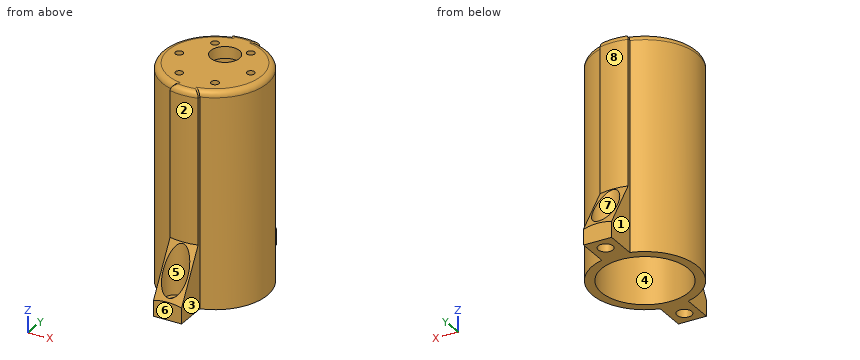
from build123d import *

# Parameters (mm, degrees)
F1_R      = 3.15
F2_DEPTH  = 92
F3_R      = 18.6
F5_DEPTH  = 87
F4_R      = 6.15
F4_R_2    = 1.65
F8_DEPTH  = 92.0010001
F9_R      = 5.25
F10_DEPTH = 87
F11_R     = 2.5


with BuildPart() as f2:
    # F1 (on Top) → F2 (new body)
    with BuildSketch(Plane.XY):
        with BuildLine():
            Line((6, 35.2), (-6, 35.2))
            Line((-6, 35.2), (-6, 21.6852484422))
            ThreePointArc((-6, 21.6852484422), (0, 22.5), (6, 21.6852484422))
            Line((6, 21.6852484422), (6, 35.2))
        make_face()
        with Locations((0, 29.2)):
            Circle(F1_R, mode=Mode.SUBTRACT)
        with BuildLine():
            ThreePointArc((6, 21.6852484422), (0, 22.5), (-6, 21.6852484422))
            ThreePointArc((-6, 21.6852484422), (-22.5, 0), (-6, -21.6852484422))
            ThreePointArc((-6, -21.6852484422), (0, -22.5), (6, -21.6852484422))
            ThreePointArc((6, -21.6852484422), (17.9060045795, -13.6244265934), (22.5, 0))
            ThreePointArc((22.5, 0), (17.9060045795, 13.6244265934), (6, 21.6852484422))
        make_face()
        with BuildLine():
            ThreePointArc((6, -21.6852484422), (0, -22.5), (-6, -21.6852484422))
            Line((-6, -21.6852484422), (-6, -35.2))
            Line((-6, -35.2), (6, -35.2))
            Line((6, -35.2), (6, -21.6852484422))
        make_face()
        with Locations((0, -29.2)):
            Circle(F1_R, mode=Mode.SUBTRACT)
    extrude(amount=F2_DEPTH)

    # F3 (on face) → F5 (cut)
    with BuildSketch(Plane(origin=(0, 0, 0), x_dir=(1, 0, 0), z_dir=(0, 0, -1))):
        Circle(F3_R)
    extrude(amount=-F5_DEPTH, mode=Mode.SUBTRACT)

    # F6 (on Right) → F7 (revolve, cut)
    with BuildSketch(Plane.YZ):
        Polygon((36.6852484422, 102), (23.6852484422, 102), (23.6852484422, 27.5166604984), (36.6852484422, 5), align=None)
    revolve(axis=Axis((0, 0, 51.2388907373), (0, 0, 1)), mode=Mode.SUBTRACT)

    # F4 (on face) → F8 (cut, through all)
    with BuildSketch(Plane.XY.offset(92)):
        with Locations((0, 7.5)):
            Circle(F4_R)
        with Locations((-15.3, 0)):
            Circle(F4_R_2)
        with Locations((-7.65, -13.2501886779)):
            Circle(F4_R_2)
        with Locations((7.65, -13.2501886779)):
            Circle(F4_R_2)
        with Locations((15.3, 0)):
            Circle(F4_R_2)
        with Locations((7.65, 13.2501886779)):
            Circle(F4_R_2)
        with Locations((-7.65, 13.2501886779)):
            Circle(F4_R_2)
    extrude(amount=-F8_DEPTH, mode=Mode.SUBTRACT)

    # F9 (on face) → F10 (cut)
    with BuildSketch(Plane.XY.offset(92)):
        with Locations((0, 29.2)):
            Circle(F9_R)
        with Locations((0, -29.2)):
            Circle(F9_R)
    extrude(amount=-F10_DEPTH, mode=Mode.SUBTRACT)

    # F11
    f11_edges = [f2.edges().sort_by_distance(p)[0] for p in [
        (-22.5, 0, 92),
        (-6, -22.298965, 92),
        (0, 23.685248, 92),
        (0, -23.685248, 92),
        (6, -22.298965, 92),
        (22.5, 0, 92),
        (6, 22.298965, 92),
        (-6, 22.298965, 92),
    ]]
    fillet(f11_edges, radius=F11_R)


solid = f2.part
For this review, take the finished solid that the model builds, in its own axes (mm). Face numbers are marked on the shaded views. A direction names the side the tool comes from. Round coordinates to 2 decimals unless told otherwise and drop trailing zeros. Write each loop counter-clockwise with the first axis right and the second up, starting at its lowest first coordinate (ties: lowest second). Pieces come first, ordered by that corner, then holes. Notation, with made-up numbers: (47.5, -29) -> (103.5, -29) arc R16 cw to (103.5, -13) -> close; hole circle Ø8 at (-28, 78). An arc over 180 degrees is marked (long way). Use CSV: the item, a comma, the result in double quotes.
(1) Consider section B-B, the plane x = 0. Give the number of separate pieces and of enclosed holes in the cut face, plus the area to 3 significant figures.
Computed values:
separate pieces,"4"
enclosed holes,"0"
area,"1,130 mm²"
(2) Consider section D-D, the plane z = 10. Give the boundary of the cut face in (x, y).
Computed values:
outline,"(-6, -33.26) arc R33.8 ccw to (-2.72, -33.69) arc R5.25 cw (long way) to (2.72, -33.69) arc R33.8 ccw to (6, -33.26) -> (6, -21.69) arc R22.5 ccw to (6, 21.69) -> (6, 33.26) arc R33.8 ccw to (2.72, 33.69) arc R5.25 cw (long way) to (-2.72, 33.69) arc R33.8 ccw to (-6, 33.26) -> (-6, 21.69) arc R22.5 ccw to (-6, -21.69) -> close; hole circle Ø37.2 at (0, 0)"
(3) For the marked faces 1, 2, 3 and 4, list the 3-axis set-ups (+Z, -Z, +X, -X, +Y, -Y) from which the entire face can be reached by the end or side of a thin tool; tool diameter is ignored.
Computed values:
face 1,"+Z, -Z, -X, +Y"
face 2,"+Z, -Y"
face 3,"+Z, -Z, +X, -Y"
face 4,"-Z"
(4) Draft analysis for pull direction X (two halves, no side actions). For the marked faces 5, 6, 7 and 8, state which applies: +X half, -X half, draft (parallel to the pull), parting line (faces both ways), or undercut.
Computed values:
face 5,"undercut"
face 6,"draft"
face 7,"undercut"
face 8,"parting line"
(5) To check wall thickness, follow L1, parallel to X at y = -0.5, z = 11; L2, parallel to Y at x = 0, z = 15; L3, parallel to X at y = 29.2, z = 11.25. State the ranges of each line that lie inside material, in increasing order. Write a range as [from, to].
Computed values:
L1,"[-22.49, -18.59], [18.59, 22.49]"
L2,"[-23.95, -18.6], [18.6, 23.95]"
L3,"[-6, -5.25], [5.25, 6]"
(6) Consider section A-A, the plane z = 37.5. Give the boundary of the cut face in (x, y).
Computed values:
outline,"(-6, -22.91) arc R23.69 ccw to (6, -22.91) -> (6, -21.69) arc R22.5 ccw to (6, 21.69) -> (6, 22.91) arc R23.69 ccw to (-6, 22.91) -> (-6, 21.69) arc R22.5 ccw to (-6, -21.69) -> close; hole circle Ø37.2 at (0, 0)"
(7) Clearance check with flat-ended pins moving along their axes: P1, Ø8, axis at y = 4, z = 80, coming from the -X side; P2, Ø8, axis at x = 1.5, z = 40, coming from the +Y side; P3, Ø1, axis at y = 21, z = 43, coming from the -X side. State where each tip first meets the part, or that it passes through.
Computed values:
P1,"x = -22.5"
P2,"y = 23.69"
P3,"x = -9.27"
